```python
from build123d import *

# Parameters (mm, degrees)
F0_R     = 31.75
F1_DEPTH = 2.9718
F2_R     = 6.0325
F2_W     = 2.9718
F2_H     = 19.05
F2_R_2   = 1.397
F3_DEPTH = 2.9718


with BuildPart() as f1:
    # F0 (on Top) → F1 (new body)
    with BuildSketch(Plane.XY):
        Circle(F0_R)
    extrude(amount=-F1_DEPTH)

    # F2 (on face) → F3 (cut, through all)
    with BuildSketch(Plane.XY):
        Circle(F2_R)
        with Locations((0, 19.05)):
            Rectangle(F2_W, F2_H)
        Polygon((-7.505942, -6.049327), (-8.991842, -3.475673), (-25.489626, -13.000673), (-24.003726, -15.574327), align=None)
        Polygon((8.991842, -3.475673), (7.505942, -6.049327), (24.003726, -15.574327), (25.489626, -13.000673), align=None)
        with Locations((-16.497784, 9.525)):
            Circle(F2_R_2)
        with Locations((16.497784, 9.525)):
            Circle(F2_R_2)
        with Locations((0, -19.05)):
            Circle(F2_R_2)
    extrude(amount=-F3_DEPTH, mode=Mode.SUBTRACT)


solid = f1.part
```
Could you check a few things on this model? Use its own coordinates, in mm. A direction names the side the tool comes from. Coordinates: 2 decimals unless noted, no trailing zeros. Order: outer loops, then holes, each group sorted by start corner. A loop starts at its lowest first (then second) coordinate and runs counter-clockwise, first axis right, second up. Notation, with made-up numbers: M -2.5,33 L 41.5,33 A22 ccw 41.5,68 Z; hole C 63,77.5 d2. An arc over 180 degrees is marked long. Use one line per item in the form item = value. Start each with the question number.
1. Suppose I cut it at D-D on y = 0. Write out the boundary of the cut face in (x, z).
2. For pin 1 (0.9 mm diameter, centred on x = -0.5, z = -2, fed in from -Y); pin 2 (1.5 mm diameter, centred on y = 14.5, z = -2, fed in from -X); pin 3 (0.9 mm diameter, centred on y = 20, z = -1.5, fed in from +X), each with a flat end and sliding along its axis, tell me the tip position at first contact or that it passes through.
3. Suppose I cut it at A-A on x = 0. Count the separate pieces of the cut face and the enclosed holes in it, then the cut area to 3 significant figures.
4. On a 3-axis mill with a long thin cutter (end or side, diameter ignored), from which of +Z, -Z, +X, -X, +Y, -Y can I reach the whole of each face in a straight line? I mean faces 1 (the flat face through (0, -7, 0)), 2 (the flat face through (24.736, -14.306, -1.465)). Say none if no direction works.
5. We'd pull the mould along X, two halves only. Please class faces 3 (the flat face through (0, 9.525, -1)), 4 (the flat face through (0, -7, -2.972)), 5 (the cylindrical face through (15.5, 10.5, -1.5)): +X half, -X half, draft (parallel to the pull), parting line (faces both ways), or undercut.
6. Please list where these lines run through material, in increasing order: line 1 (X direction, y = -6.5, z = -1.3); line 2 (X direction, y = -13.5, z = -2.55); line 3 (Y direction, x = -22.5, z = -0.8).
7. Suppose I cut it at B-B on y = -19.05. Write out the boundary of the cut face in (x, z), then the cut area to 3 significant figures.
Geometry says:
q1.outline = M -31.75,-2.97 L -6.03,-2.97 L -6.03,0 L -31.75,0 Z; M 6.03,-2.97 L 31.75,-2.97 L 31.75,0 L 6.03,0 Z
q2.pin_1 = -31.75
q2.pin_2 = -28.62
q2.pin_3 = 25.02
q3.separate_pieces = 4
q3.enclosed_holes = 0
q3.area = 87.9 mm^2
q4.face_1 = +Z, +X, -X, +Y, -Y
q4.face_2 = +Z, -Z
q5.face_3 = undercut
q5.face_4 = draft
q5.face_5 = undercut
q6.line_1 = -31.08 to -14.23, -8.29 to 8.29, 14.23 to 31.08
q6.line_2 = -28.74 to -25.2, -20.41 to 20.41, 25.2 to 28.74
q6.line_3 = -22.4 to -14.71, -11.27 to 22.4
q7.outline = M -25.4,-2.97 L -1.4,-2.97 L -1.4,0 L -25.4,0 Z; M 1.4,-2.97 L 25.4,-2.97 L 25.4,0 L 1.4,0 Z
q7.area = 143 mm^2
